Could you check a few things on this model? Use its own coordinates, in mm. Face numbers are marked on the shaded views. A direction names the side the tool comes from. Give positions to 0.01 mm unless a question says otherwise; leave off trailing zeros. Write each loop counter-clockwise with the first axis right and the second up, starting at its lowest first coordinate (ties: lowest second). Pieces come first, ordered by that corner, then holes. Notation, with made-up numbers: M -13.75,86.25 L 2.25,86.25 A20 cw 2.25,91.25 Z; hole C -12,-38.75 d5. An arc over 180 degrees is marked long. Use one line per item in the form item = value.
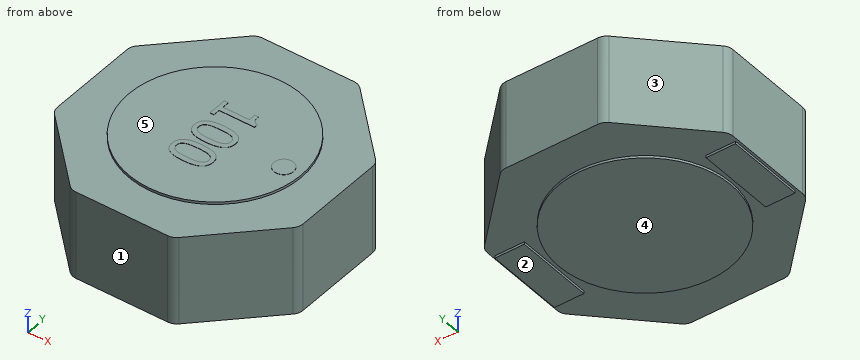
Autodesk Inventor part; units mm, degrees
ref_plane "YZ Plane" through (0, 0, 0) normal (1, 0, 0) x (0, 1, 0)
ref_plane "XZ Plane" through (0, 0, 0) normal (0, 1, 0) x (-1, 0, 0)
ref_plane "XY Plane" through (0, 0, 0) normal (0, 0, 1) x (1, 0, 0)
sketch "Sketch1" plane through (0, 0, 0) normal (0, 0, 1) x (1, 0, 0)
  circle A0 centre (0, 0) radius 3.5
  dimension "d0" = 7
extrude "Extrusion1" add sketch "Sketch1" along normal mid plane 3.8
sketch "Sketch2" plane through (0, 0, 0) normal (0, 0, 1) x (1, 0, 0)
  line L0 (2.0711, 5) -> (5, 2.0711)
  line L1 (5, 2.0711) -> (5, -2.0711)
  line L2 (5, -2.0711) -> (2.0711, -5)
  line L3 (2.0711, -5) -> (-2.0711, -5)
  line L4 (-2.0711, -5) -> (-5, -2.0711)
  line L5 (-5, -2.0711) -> (-5, 2.0711)
  line L6 (-5, 2.0711) -> (-2.0711, 5)
  line L7 (-2.0711, 5) -> (2.0711, 5)
  point P0 (0, 0)
  point P1 (0, 0)
  dimension "d3" = 10
extrude "Extrusion2" add sketch "Sketch2" along normal mid plane 3.6
sketch "Sketch3" plane through (0, 0, -1.8) normal (0, 0, -1) x (-1, 0, 0)
  line L0 (-2.0711, 5) -> (-5, 2.0711)
  line L1 (-5, 2.0711) -> (-5, -2.0711)
  line L2 (-5, -2.0711) -> (-2.0711, -5)
  line L3 (-2.0711, -5) -> (2.0711, -5)
  line L4 (2.0711, -5) -> (5, -2.0711)
  line L5 (5, -2.0711) -> (5, 2.0711)
  line L6 (5, 2.0711) -> (2.0711, 5)
  line L7 (2.0711, 5) -> (-2.0711, 5)
  circle A0 centre (0, 0) radius 3.5
  line L8 (-4.9, -1.6) -> (-3.7, -1.6)
  line L9 (-3.7, -1.6) -> (-3.7, 1.6)
  line L10 (-3.7, 1.6) -> (-4.9, 1.6)
  line L11 (-4.9, 1.6) -> (-4.9, -1.6)
  line L12 (4.9, -1.6) -> (3.7, -1.6)
  line L13 (3.7, -1.6) -> (3.7, 1.6)
  line L14 (3.7, 1.6) -> (4.9, 1.6)
  line L15 (4.9, 1.6) -> (4.9, -1.6)
  point P0 (-4.9, 0)
  point P1 (-5, 0)
  dimension "d6" = 3.2
  dimension "d7" = 0.1
  dimension "d8" = 0.1
  dimension "d9" = 7.4
extrude "Extrusion3" add sketch "Sketch3" along normal blind 0.1 contours L11 L10 L9 L8 | L12 L13 L14 L15
sketch "Sketch4" plane through (0, 0, 1.9) normal (0, 0, 1) x (1, 0, 0)
  circle A0 centre (0, 0) radius 3.5
  circle A1 centre (2.8, 0) radius 0.4
  circle A2 centre (0, 0) radius 3.5 construction
  line L0 (0, 3.5) -> (0, -3.5) construction
  line L1 (-0.8, 0.778) -> (-0.8, 1.5585)
  line L2 (-0.8, 1.5585) -> (-0.6366, 1.5585)
  line L3 (-0.6366, 1.5585) -> (-0.6366, 1.2681)
  line L4 (-0.6366, 1.2681) -> (0.4357, 1.2681)
  line L5 (0.4357, 1.2681) -> (0.4357, 1.5585)
  line L6 (0.4357, 1.5585) -> (0.5822, 1.5585)
  spline S0 degree 2 poles (0.5822, 1.5585) (0.5822, 1.3938) (0.6755, 1.2382) (0.8052, 1.2279) knots 0 0 0 1 2 2 2
  line L7 (0.8052, 1.2279) -> (0.8052, 1.0619)
  line L8 (0.8052, 1.0619) -> (-0.6366, 1.0619)
  line L9 (-0.6366, 1.0619) -> (-0.6366, 0.778)
  line L10 (-0.6366, 0.778) -> (-0.8, 0.778)
  spline S1 degree 2 poles (0, -0.5122) (-0.4305, -0.5122) (-0.8337, -0.2619) (-0.8337, -0.0013) knots 0 0 0 1 2 2 2
  spline S2 degree 2 poles (-0.8337, -0.0013) (-0.8337, 0.2632) (-0.4227, 0.5109) (-0.0013, 0.5109) knots 0 0 0 1 2 2 2
  spline S3 degree 2 poles (-0.0013, 0.5109) (0.4318, 0.5109) (0.8324, 0.2606) (0.8324, -0.0013) knots 0 0 0 1 2 2 2
  spline S4 degree 2 poles (0.8324, -0.0013) (0.8324, -0.2645) (0.4175, -0.5122) (0, -0.5122) knots 0 0 0 1 2 2 2
  spline S5 degree 2 poles (-0.4875, -0.2373) (-0.4084, -0.2684) (-0.1647, -0.2943) (0, -0.2943) knots 0 0 0 1 2 2 2
  spline S6 degree 2 poles (0, -0.2943) (0.1647, -0.2943) (0.4071, -0.2684) (0.4888, -0.236) knots 0 0 0 1 2 2 2
  spline S7 degree 2 poles (0.4888, -0.236) (0.5705, -0.2036) (0.6548, -0.0908) (0.6548, -0.0013) knots 0 0 0 1 2 2 2
  spline S8 degree 2 poles (0.6548, -0.0013) (0.6548, 0.0882) (0.5705, 0.2036) (0.4862, 0.2373) knots 0 0 0 1 2 2 2
  spline S9 degree 2 poles (0.4862, 0.2373) (0.4045, 0.2697) (0.1556, 0.293) (-0.0013, 0.293) knots 0 0 0 1 2 2 2
  spline S10 degree 2 poles (-0.0013, 0.293) (-0.1699, 0.293) (-0.3955, 0.2723) (-0.4836, 0.2386) knots 0 0 0 1 2 2 2
  spline S11 degree 2 poles (-0.4836, 0.2386) (-0.5666, 0.2075) (-0.6561, 0.0921) (-0.6561, -0.0013) knots 0 0 0 1 2 2 2
  spline S12 degree 2 poles (-0.6561, -0.0013) (-0.6561, -0.0895) (-0.5718, -0.2049) (-0.4875, -0.2373) knots 0 0 0 1 2 2 2
  spline S13 degree 2 poles (0, -1.7128) (-0.4305, -1.7128) (-0.8337, -1.4626) (-0.8337, -1.2019) knots 0 0 0 1 2 2 2
  spline S14 degree 2 poles (-0.8337, -1.2019) (-0.8337, -0.9374) (-0.4227, -0.6898) (-0.0013, -0.6898) knots 0 0 0 1 2 2 2
  spline S15 degree 2 poles (-0.0013, -0.6898) (0.4318, -0.6898) (0.8324, -0.94) (0.8324, -1.2019) knots 0 0 0 1 2 2 2
  spline S16 degree 2 poles (0.8324, -1.2019) (0.8324, -1.4652) (0.4175, -1.7128) (0, -1.7128) knots 0 0 0 1 2 2 2
  spline S17 degree 2 poles (-0.4875, -1.4379) (-0.4084, -1.469) (-0.1647, -1.495) (0, -1.495) knots 0 0 0 1 2 2 2
  spline S18 degree 2 poles (0, -1.495) (0.1647, -1.495) (0.4071, -1.469) (0.4888, -1.4366) knots 0 0 0 1 2 2 2
  spline S19 degree 2 poles (0.4888, -1.4366) (0.5705, -1.4042) (0.6548, -1.2914) (0.6548, -1.2019) knots 0 0 0 1 2 2 2
  spline S20 degree 2 poles (0.6548, -1.2019) (0.6548, -1.1125) (0.5705, -0.9971) (0.4862, -0.9634) knots 0 0 0 1 2 2 2
  spline S21 degree 2 poles (0.4862, -0.9634) (0.4045, -0.931) (0.1556, -0.9076) (-0.0013, -0.9076) knots 0 0 0 1 2 2 2
  spline S22 degree 2 poles (-0.0013, -0.9076) (-0.1699, -0.9076) (-0.3955, -0.9284) (-0.4836, -0.9621) knots 0 0 0 1 2 2 2
  spline S23 degree 2 poles (-0.4836, -0.9621) (-0.5666, -0.9932) (-0.6561, -1.1086) (-0.6561, -1.2019) knots 0 0 0 1 2 2 2
  spline S24 degree 2 poles (-0.6561, -1.2019) (-0.6561, -1.2901) (-0.5718, -1.4055) (-0.4875, -1.4379) knots 0 0 0 1 2 2 2
  dimension "d12" = 0.8
  dimension "d13" = 2.8
extrude "Extrusion4" add sketch "Sketch4" along normal blind 0.01 contours A1 | L1 L2 L3 L4 L5 L6 S0 L7 L8 L9 L10 | S1 S2 S3 S4 | S13 S14 S15 S16
fillet "Fillet1" radius 0.5 8 edges at (-2.0711, -5, 0) (2.0711, -5, 0) (5, -2.0711, 0) (5, 2.0711, 0) (2.0711, 5, 0) (-2.0711, 5, 0) (-5, 2.0711, 0) (-5, -2.0711, 0)
equation "\"d8\" = d7"
properties part number "34-103B" material "Iron, Cast"
1) If I drill on L1, parallel to Z at x = 0.5, y = -2; L2, parallel to Z at x = 3, y = 2.75; L3, parallel to Y at x = 3, z = 0.1, over which ranges is the centre line in solid material (lowest first)?
Checked values:
L1 = -1.9 to 1.9
L2 = -1.8 to 1.8
L3 = -4.07 to 4.07
2) For pin 1 Ø2 at (x, z) = (4, -0.5) entering from -Y, with a flat end and sliding along its axis, tell me the tip position at first contact or that it passes through.
Checked values:
pin_1 = -4.07
3) Thinking about a two-plate mould opening in Y: for the marked faces 1, 2 and 3, which applies, released by +Y, released by -Y, zero draft, split by the parting line, or undercut?
Checked values:
face_1 = released by -Y
face_2 = zero draft
face_3 = released by +Y
4) I want a section at C-C, the plane y = 2. Please give me the cut outline in (x, z).
Checked values:
outline = M -4.98,-1.8 L -2.87,-1.8 L -2.87,-1.9 L 2.87,-1.9 L 2.87,-1.8 L 4.98,-1.8 L 4.98,1.8 L 2.87,1.8 L 2.87,1.9 L -2.87,1.9 L -2.87,1.8 L -4.98,1.8 Z
5) I want a section at A-A, the plane z = 1.3. Please give me the cut outline in (x, y).
Checked values:
outline = M -5,-1.86 A0.5 ccw -4.85,-2.22 L -2.22,-4.85 A0.5 ccw -1.86,-5 L 1.86,-5 A0.5 ccw 2.22,-4.85 L 4.85,-2.22 A0.5 ccw 5,-1.86 L 5,1.86 A0.5 ccw 4.85,2.22 L 2.22,4.85 A0.5 ccw 1.86,5 L -1.86,5 A0.5 ccw -2.22,4.85 L -4.85,2.22 A0.5 ccw -5,1.86 Z
6) I want a section at B-B, the plane x = -4.25. Please give me the cut outline in (y, z), plus the area to 3 significant figures.
Checked values:
outline = M -2.82,-1.8 L -1.6,-1.8 L -1.6,-1.9 L 1.6,-1.9 L 1.6,-1.8 L 2.82,-1.8 L 2.82,1.8 L -2.82,1.8 Z
area = 20.6 mm2
7) For the marked faces 4 and 5, which set-ups out of +Z, -Z, +X, -X, +Y, -Y let a thin tool reach every point of the face, with its end or its side?
Checked values:
face_4 = -Z, +X, -X, +Y, -Y
face_5 = +Z
